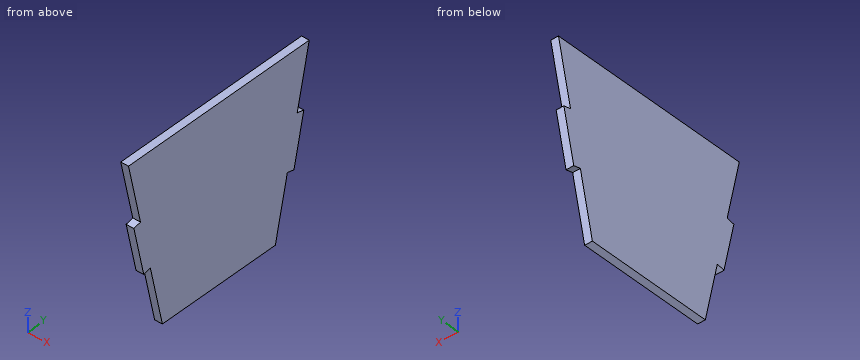
Solid Edge part; units mm, degrees
sketch "Sketch1" plane through (0, 0, 0) normal (1, 0, 0) x (0, 1, 0)
  line L0 (40, 66.9227) -> (34.6871, 43.2192)
  line L1 (34.6871, 43.2192) -> (37.6145, 42.5631)
  line L2 (37.6145, 42.5631) -> (33.2402, 23.0473)
  line L3 (33.2402, 23.0473) -> (30.3129, 23.7035)
  line L4 (30.3129, 23.7035) -> (25, 0)
  line L5 (25, 0) -> (-25, 0)
  line L6 (-25, 0) -> (-30.3129, 23.7035)
  line L7 (-30.3129, 23.7035) -> (-33.2402, 23.0473)
  line L8 (-33.2402, 23.0473) -> (-37.6145, 42.5631)
  line L9 (-37.6145, 42.5631) -> (-34.6871, 43.2192)
  line L10 (-34.6871, 43.2192) -> (-40, 66.9227)
  line L11 (-40, 66.9227) -> (40, 66.9227)
  dimension "D1" = 40
  dimension "D2" = 25
  dimension "D3" = 34.6871
  dimension "D4" = 37.6145
  dimension "D5" = 40
extrude "Protrusion1" add sketch "Sketch1" against normal blind 3
properties material "Acier"
Check sheet for the modelled part. Datum: model origin and axes. Units: mm. Coordinates: 2 decimals unless noted, no trailing zeros. Loops run counter-clockwise (first coordinate to the right, second up) from the corner with the lowest first, then second, coordinate; pieces in that order, holes last. Notation, with made-up numbers: (53, -18.5) -> (84, -18.5) arc R23 ccw to (84, 20.5) -> close; hole circle Ø1 at (62, 65). An arc over 180 degrees is marked (long way). Write item = value, one per line. Start each with the question number.
1. Material ranges on line 1 (Y direction, x = -2.6, z = 29.5); line 2 (Y direction, x = -1.9, z = 48); line 3 (Z direction, x = -2.4, y = 32), recorded low to high.
2. Section check C-C on y = -27. Record the cut outline in (x, z), then the cut area to 3 significant figures.
3. Section check B-B on z = 38.5. Record the cut outline in (x, y), then the cut area to 3 significant figures.
4. Section check A-A on x = -2.2. Record the cut outline in (y, z), then the cut area to 3 significant figures.
Responses:
q1.line_1 = -34.69 to 34.69
q1.line_2 = -35.76 to 35.76
q1.line_3 = 23.33 to 66.92
q2.outline = (-3, 8.92) -> (0, 8.92) -> (0, 66.92) -> (-3, 66.92) -> close
q2.area = 174 mm2
q3.outline = (-3, -36.7) -> (0, -36.7) -> (0, 36.7) -> (-3, 36.7) -> close
q3.area = 220 mm2
q4.outline = (-40, 66.92) -> (-34.69, 43.22) -> (-37.61, 42.56) -> (-33.24, 23.05) -> (-30.31, 23.7) -> (-25, 0) -> (25, 0) -> (30.31, 23.7) -> (33.24, 23.05) -> (37.61, 42.56) -> (34.69, 43.22) -> (40, 66.92) -> close
q4.area = 4,470 mm2
